Autodesk Inventor part; units mm, degrees
ref_plane "YZ Plane" through (0, 0, 0) normal (1, 0, 0) x (0, 1, 0)
ref_plane "XZ Plane" through (0, 0, 0) normal (0, 1, 0) x (-1, 0, 0)
ref_plane "XY Plane" through (0, 0, 0) normal (0, 0, 1) x (1, 0, 0)
sketch "Sketch - Bearing Body" plane through (0, 0, 0) normal (0, 0, 1) x (1, 0, 0)
  line L0 (55.8, 0) -> (55.8, 7.3)
  line L1 (55.8, 7.3) -> (0, 7.3)
  line L2 (0, 7.3) -> (0, 0)
  line L3 (38.8, 0) -> (38.8, -23)
  line L4 (17, -23) -> (17, 0)
  line L5 (17, -23) -> (-8.9808, -38)
  line L6 (-8.9808, -38) -> (1.9192, -56.8794)
  line L7 (1.9192, -56.8794) -> (27.9, -41.8794)
  line L8 (38.8, -23) -> (64.7808, -38)
  line L9 (64.7808, -38) -> (53.8808, -56.8794)
  line L10 (53.8808, -56.8794) -> (27.9, -41.8794)
  line L11 (0, 0) -> (17, 0)
  line L12 (38.8, 0) -> (55.8, 0)
  line L13 (24.3, 0) -> (31.5, 0)
  line L14 (31.5, 0) -> (31.5, -22.9717)
  line L15 (24.3, -22.9717) -> (24.3, 0)
  line L16 (0.9912, -40.672) -> (4.5912, -46.9074)
  line L17 (4.5912, -46.9074) -> (24.077, -35.6572)
  line L18 (0.9912, -40.672) -> (20.55, -29.3797)
  line L19 (51.2088, -46.9074) -> (54.8088, -40.672)
  line L20 (54.8088, -40.672) -> (35.25, -29.3797)
  line L21 (51.2088, -46.9074) -> (31.723, -35.6572)
  circle A0 centre (27.9, -29.3797) radius 7.35
  point P0 (17, -11.5)
  point P1 (51.7904, -30.5)
  dimension "d1" = 7.3
  dimension "d3" = 23
  dimension "LegLength" = 30
  dimension "d7" = 21.8
  dimension "d12" = 30
  dimension "d13" = 21.8
  dimension "LegAngle2" = 120
  dimension "d15" = 120
  dimension "d17" = 21.8
  dimension "d19" = 17
  dimension "d20" = 17
  dimension "d22" = 7.2
  dimension "d23" = 7.3
  dimension "d24" = 7.3
  dimension "d25" = 7.2
  dimension "d26" = 7.3
  dimension "d27" = 7.2
  dimension "d28" = 7.3
  dimension "d29" = 7.3
  dimension "d77" = 14.7
extrude "Extrusion - Bearing Body" add sketch "Sketch - Bearing Body" along normal blind 60
sketch "Sketch - Bearing Screw Holes 1" plane through (17, -23, 60) normal (-0.5, 0.866, 0) x (0.866, 0.5, 0)
  line L0 (-30, 0) -> (0, 0)
  line L1 (-30, 60) -> (0, 60)
  line L2 (-30, 60) -> (-30, 0)
  line L3 (0, 60) -> (0, 0)
  line L4 (-12.1, 48.2) -> (-10.1, 48.2)
  line L5 (-12.1, 39.8) -> (-10.1, 39.8)
  line L6 (-12.1, 20.2) -> (-10.1, 20.2)
  line L7 (-12.1, 11.8) -> (-10.1, 11.8)
  arc A0 (-12.1, 20.2) -> (-12.1, 11.8) centre (-12.1, 16) ccw
  arc A1 (-10.1, 11.8) -> (-10.1, 20.2) centre (-10.1, 16) ccw
  arc A2 (-10.1, 39.8) -> (-10.1, 48.2) centre (-10.1, 44) ccw
  arc A3 (-12.1, 48.2) -> (-12.1, 39.8) centre (-12.1, 44) ccw
  point P0 (-3.2224, 60)
  point P1 (-11.1, 16)
  point P2 (-11.1, 44)
  point P3 (-11.1, 48.2)
  point P4 (-11.1, 39.8)
  point P5 (-11.1, 20.2)
  point P6 (-11.1, 11.8)
  dimension "d47" = 16
  dimension "d48" = 18.9
  dimension "d49" = 16
  dimension "BearingHoleElipseMiddle" = 2
  dimension "BearingBoltRadius" = 4.2
  dimension "d91" = 4.2
  dimension "d92" = 4.2
  dimension "d93" = 4.2
  dimension "d94" = 4.2
sketch "Sketch - Bearing Screw Holes 2" plane through (64.7808, -38, 60) normal (0.5, 0.866, 0) x (0.866, -0.5, 0)
  line L0 (-30, 0) -> (0, 0)
  line L1 (0, 60) -> (0, 0)
  line L2 (-30, 60) -> (0, 60)
  point P0 (-75.1018, 60)
  point P1 (-18.9, 16)
  point P2 (-18.9, 44)
  dimension "d50" = 18.9
  dimension "d51" = 16
  dimension "d52" = 16
hole "Hole - Bearing Screw Holes 2" at (48.4129, -28.55, 16) at (48.4129, -28.55, 44) direction (-0.5, -0.866, 0) diameter 9 end through all
sketch "Sketch - Bearing Screw Holes 3" plane through (17, -23, 0) normal (-1, 0, 0) x (0, 0, 1)
  line L0 (60, 0) -> (60, 23)
  line L1 (0, 23) -> (60, 23)
  line L2 (0, 0) -> (0, 23)
  point P0 (16, 10.97)
  point P1 (44, 10.97)
  dimension "d67" = 16
  dimension "d68" = 12.03
  dimension "d69" = 16
hole "Hole - Bearing Screw Holes 3" at (17, -12.03, 16) at (17, -12.03, 44) direction (1, 0, 0) diameter 8 end through all
sketch "Sketch - Plate Holes" plane through (0, 7.3, 0) normal (0, 1, 0) x (1, 0, 0)
  line L0 (0, -60) -> (55.8, -60)
  line L1 (55.8, 0) -> (55.8, -60)
  line L2 (0, 0) -> (55.8, 0)
  line L3 (0, 0) -> (0, -60)
  point P0 (8, -16)
  point P1 (8, -44)
  point P2 (47.8, -16)
  point P3 (47.8, -44)
  dimension "PlateAttachmentHoleVert" = 16
  dimension "d79" = 16
  dimension "PlateAttachmentHoleHoriz" = 8
  dimension "d81" = 8
hole "Hole - Plate Holes" at (8, 7.3, 16) at (8, 7.3, 44) at (47.8, 7.3, 16) at (47.8, 7.3, 44) direction (0, -1, 0) diameter 3.797 depth 7.3 tip angle 118
extrude "Extrusion4" cut sketch "Sketch - Bearing Screw Holes 1" against normal through all contours L4 A2 L5 A3 | L6 A1 L7 A0
sketch "Sketch7" plane through (-8.9808, -38, 0) normal (-0.866, -0.5, 0) x (0, 0, 1)
  line L0 (60, -21.8) -> (60, 0)
  line L1 (0, 0) -> (60, 0)
  line L2 (0, -21.8) -> (0, 0)
  line L3 (0, -21.8) -> (60, -21.8)
  point P0 (0, 28.4186)
  point P1 (16, -3.65)
  point P2 (16, -18.15)
  point P3 (44, -18.15)
  point P4 (44, -3.65)
  dimension "d97" = 3.65
  dimension "d98" = 3.65
  dimension "d99" = 16
  dimension "d100" = 16
hole "Hole5" at (-7.1558, -41.161, 16) at (0.0942, -53.7184, 16) at (0.0942, -53.7184, 44) at (-7.1558, -41.161, 44) direction (0.866, 0.5, 0) diameter 2.642 depth 15
equation "\"d1\" = WallWidth"
equation "\"d7\" = SupportWidth"
equation "\"d12\" = LegLength"
equation "\"d13\" = SupportWidth"
equation "\"LegAngle2\" = LegAngle"
equation "\"d15\" = LegAngle"
equation "\"d17\" = SupportWidth"
equation "\"d19\" = PlateHangOver"
equation "\"d20\" = PlateHangOver"
equation "\"d22\" = BearingWidth + BearingPadding"
equation "\"d23\" = WallWidth"
equation "\"d24\" = WallWidth"
equation "\"d25\" = BearingWidth + BearingPadding"
equation "\"d26\" = WallWidth"
equation "\"d27\" = BearingWidth + BearingPadding"
equation "\"d28\" = WallWidth"
equation "\"d29\" = WallWidth"
equation "\"d94\" = 0.5 * BearingHoleSize"
equation "\"d87\" = WallWidth"
equation "\"LegAngle\" = 120deg"
equation "\"BearingWidth\" = 7"
equation "\"BearingOuterDiameter\" = 22"
equation "\"BearingPadding\" = 0.2"
equation "\"SupportWidth\" = BearingWidth + 2 * WallWidth + BearingPadding"
equation "\"PlateHangOver\" = 17"
equation "\"RodDiameter\" = 12.7"
equation "\"RodDiameterPadding\" = 2"
equation "\"WallWidth\" = 7.3"
equation "\"BearingHoleSize\" = 8.4"
properties part number "LinearBearing"
The listing builds one solid part. Answer for the finished solid, in the listing's coordinates (mm). A direction names the side the tool comes from. Coordinates: 2 decimals unless noted, no trailing zeros. Write each loop counter-clockwise with the first axis right and the second up, starting at its lowest first coordinate (ties: lowest second). Pieces come first, ordered by that corner, then holes. Notation, with made-up numbers: M 23.25,-35.5 L 74.25,-35.5 A11 cw 74.25,-21.5 Z; hole C -10.75,34.5 d4. An arc over 180 degrees is marked long. Use a Markdown table: item, result. Add a question column.
1. Section C-C (x = 29.5) is taken. Give the vertices of the cut face in (y, z).
2. Section A-A (z = 10) is taken. Give the vertices of the cut face in (x, y).
3. Given P1, Ø1.5, axis at y = -5, z = 31, coming from the -X side; P2, Ø8, axis at y = 3, z = 22.5, coming from the +X side; P3, Ø4, axis at y = -1.5, z = 17, coming from the -X side; P4, Ø7, axis at y = -12.03, z = 16, coming from the -X side, each flat-ended and moving along its own axis, determine where each tip first touches the part or whether it passes through.
4. Section D-D (y = -24.5) is taken. Give the vertices of the cut face in (x, z).
5. For a pull along Y with two mould halves and no side action, classify faces 1 (the flat face through (55.8, 4, 30)), 2 (the cylindrical face through (6.46, -50.63, 42.78)) as +Y half, -Y half, draft (parallel to the pull), parting line (faces both ways), or undercut.
6. Section B-B (y = -12.03) is taken. Give the vertices of the cut face in (x, z), plus the area to 3 significant figures.
7. Which of the six approach directions +Z, -Z, +X, -X, +Y, -Y give full straight-line access (tool end or side, diameter ignored) to faces 3 (the flat face through (51.609, -30.395, 29.58)), 4 (the flat face through (9, -32, 48.2)), 5 (the flat face through (2.77, -43.75, 29.58))?
8. Straight lines are drawn through the part: line 1 along Z through (x, y) = (33.75, -12.03); line 2 along Z through (x, y) = (47.8, 2.5); line 3 along X through (y, z) = (-22.5, 23.5). For each, find the intervals that lie inside material, in ascending order. Write a range as [from, to].
Data:
| question | item | result |
|---|---|---|
| 1 | outline | M -42.8,0 L -36.55,0 L -36.55,60 L -42.8,60 Z; M 0,0 L 7.3,0 L 7.3,60 L 0,60 Z |
| 2 | outline | M -8.98,-38 L 1.92,-56.88 L 27.9,-41.88 L 53.88,-56.88 L 64.78,-38 L 38.8,-23 L 38.8,0 L 55.8,0 L 55.8,7.3 L 0,7.3 L 0,0 L 17,0 L 17,-23 Z; hole M 0.99,-40.67 L 4.59,-46.91 L 24.08,-35.66 A7.35 ccw 31.72,-35.66 L 51.21,-46.91 L 54.81,-40.67 L 35.25,-29.38 A7.35 ccw 31.5,-22.97 L 31.5,0 L 24.3,0 L 24.3,-22.97 A7.35 ccw 20.55,-29.38 Z |
| 3 | P1 | stops at x = 17 |
| 3 | P2 | stops at x = 55.8 |
| 3 | P3 | stops at x = 0 |
| 3 | P4 | passes through |
| 4 | outline | M 14.4,0 L 22.4,0 L 22.4,60 L 14.4,60 Z; M 33.4,0 L 41.4,0 L 41.4,60 L 33.4,60 Z |
| 5 | face 1 | draft |
| 5 | face 2 | undercut |
| 6 | outline | M 17,0 L 24.3,0 L 24.3,12 L 17,12 Z; M 17,20 L 24.3,20 L 24.3,40 L 17,40 Z; M 17,48 L 24.3,48 L 24.3,60 L 17,60 Z; M 31.5,0 L 38.8,0 L 38.8,12 L 31.5,12 Z; M 31.5,20 L 38.8,20 L 38.8,40 L 31.5,40 Z; M 31.5,48 L 38.8,48 L 38.8,60 L 31.5,60 Z |
| 6 | area | 642 mm2 |
| 7 | face 3 | +Z, -Z, +X |
| 7 | face 4 | none |
| 7 | face 5 | +Z, -Z |
| 8 | line 1 | z = [0, 12], [20, 40], [48, 60] |
| 8 | line 2 | z = [0, 14.1], [17.9, 42.1], [45.9, 60] |
| 8 | line 3 | x = [17, 24.3], [31.5, 38.8] |
